Input: part model. Units: mm. Frame: model coordinates. Face numbers are marked on the shaded views. A direction names the side the tool comes from. Coordinates: 2 decimals unless noted, no trailing zeros. Loops run counter-clockwise (first coordinate to the right, second up) from the corner with the lowest first, then second, coordinate; pieces in that order, holes last.
(1) Set-up query: the marked faces 5, 6 and 7. Return all of +Z, -Z, +X, -X, +Y, -Y with unobstructed straight access to the full face (end or side cutting, diameter ignored); none if empty.
(2) Section D-D, the plane x = 6.5. Return loops of the section in (y, z).
(3) Section A-A, the plane x = 0. Return loops of the section in (y, z) (3 decimals).
(4) Line query: L1, parallel to X at y = -4.75, z = 3; L2, parallel to Z at x = 9.25, y = -2.5; L3, parallel to Z at x = 0, y = -4 (3 decimals). Output: solid intervals per line, ascending.
(5) Contact query for flat-ended pins moving along their axis: P1, Ø2.5, axis at x = 15.5, y = -3.5, coming from the +Z side; P2, Ø2.5, axis at x = 13, y = -6, coming from the -Z side; P3, Ø1, axis at y = -4.5, z = 5.5, coming from the -X side. Output: stop coordinate, or through.
(6) Mould query, pull axis X, two halves, no side actions, for the marked faces 1, 2, 3 and 4. Classes: released by +X, released by -X, zero draft, split by the parting line, or undercut.
(7) Section C-C, the plane y = -1.25. Return loops of the section in (x, z) (3 decimals), then the cut area to 3 significant figures.
(8) Section B-B, the plane z = 2.75. Give the number of separate pieces and of enclosed holes in the cut face, then the cut area to 3 significant figures.
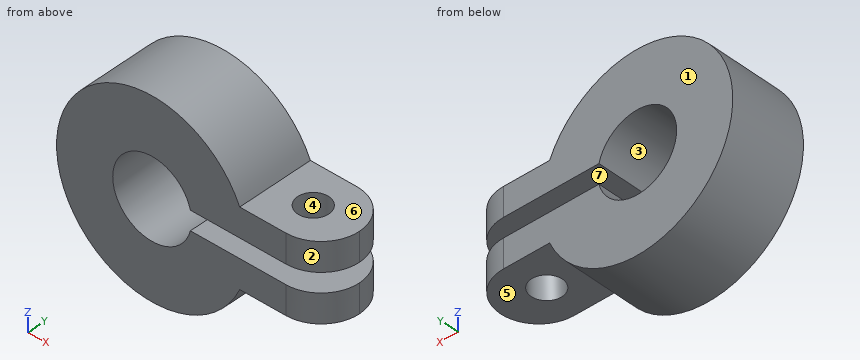
```python
from build123d import *

# Parameters (mm, degrees)
F1_DEPTH = 8
F2_R     = 1.625
F3_DEPTH = 14.001
F4_R     = 3.99999


# Not quite as in the source:
# - a fillet or chamfer is up to 0.001 mm smaller than in the source, because OpenCascade refuses the exact size


with BuildPart() as f1:
    # F0 (on Front) → F1 (new body)
    with BuildSketch(Plane.XZ):
        with BuildLine():
            ThreePointArc((4.0019526484, -1), (-4.125, 0), (4.0019526484, 1))
            Line((4.0019526484, 1), (18, 1))
            Line((18, 1), (18, 4))
            Line((18, 4), (9.1651513899, 4))
            ThreePointArc((9.1651513899, 4), (-10, 0), (9.1651513899, -4))
            Line((9.1651513899, -4), (18, -4))
            Line((18, -4), (18, -1))
            Line((18, -1), (4.0019526484, -1))
        make_face()
    extrude(amount=F1_DEPTH)

    # F2 (on face) → F3 (cut, through all)
    with BuildSketch(Plane.XY.offset(4)):
        with Locations((13.1651513899, -4.0000034496)):
            Circle(F2_R)
    extrude(amount=-F3_DEPTH, mode=Mode.SUBTRACT)

    # F4 (radius 4 in the source; OpenCascade refuses exactly that, so slightly less here)
    f4_edges = [f1.edges().sort_by_distance(p)[0] for p in [
        (18, -8, 2.5),
        (18, -8, -2.5),
        (18, 0, -2.5),
        (18, 0, 2.5),
    ]]
    fillet(f4_edges, radius=F4_R)


solid = f1.part
```
Report:
1. face 5: -Z, +X, +Y, -Y
1. face 6: +Z, +X, +Y, -Y
1. face 7: +X, +Y, -Y
2. outline: (-8, -7.6) - (0, -7.6) - (0, -1) - (-8, -1) - close; (-8, 1) - (0, 1) - (0, 7.6) - (-8, 7.6) - close
3. outline: (-8, -10) - (0, -10) - (0, -4.125) - (-8, -4.125) - close; (-8, 4.125) - (0, 4.125) - (0, 10) - (-8, 10) - close
4. L1: x = -9.54 to -2.83, 2.83 to 11.72, 14.61 to 17.93
4. L2: z = -4 to -1, 1 to 4
4. L3: z = -10 to -4.125, 4.125 to 10
5. P1: stops at z = 4
5. P2: stops at z = -4
5. P3: stops at x = -8.66
6. face 1: zero draft
6. face 2: released by +X
6. face 3: undercut
6. face 4: undercut
7. outline: (4.002, -1) arc R4.125 cw (long way) to (4.002, 1) - (16.905, 1) - (16.905, 4) - (9.165, 4) arc R10 ccw (long way) to (9.165, -4) - (16.905, -4) - (16.905, -1) - close
7. area: 292 mm2
8. separate pieces: 2
8. enclosed holes: 1
8. area: 157 mm2
